Source: CAD feature listing. Evaluate the final solid. Frame: model axes, mm. A direction names the side the tool comes from. Give positions to 0.01 mm unless a question says otherwise; leave off trailing zeros. Order: outer loops, then holes, each group sorted by start corner. A loop starts at its lowest first (then second) coordinate and runs counter-clockwise, first axis right, second up.
from build123d import *

# Parameters (mm, degrees)
ESQUISSE1_W             = 34.9
ESQUISSE1_H             = 3
BOSS_EXTRU_1_DEPTH      = 50
ESQUISSE2_W             = 10
ESQUISSE2_H             = 3.5
BOSS_EXTRU_2_DEPTH      = 9.2
ESQUISSE3_R             = 2.2
BOSS_EXTRU_3_DEPTH      = 4.5
CONG_1_R                = 0.5
ESQUISSE5_W             = 4.7
ESQUISSE5_H             = 2.5
BOSS_EXTRU_5_DEPTH      = 11.8
ENL_V_MAT_EXTRU_1_REACH = 29.05
ESQUISSE6_R             = 1
CONG_2_R                = 10


with BuildPart() as part:
    # Esquisse1 → Boss.-Extru.1 (new body)
    with BuildSketch(Plane.XY):
        with Locations((17.45, 1.5)):
            Rectangle(ESQUISSE1_W, ESQUISSE1_H)
    extrude(amount=BOSS_EXTRU_1_DEPTH)

    # Esquisse2 → Boss.-Extru.2 (add)
    with BuildSketch(Plane(origin=(0, 3, 0), x_dir=(1, 0, 0), z_dir=(0, 1, 0))):
        with Locations((12.1, -8.77)):
            Rectangle(ESQUISSE2_W, ESQUISSE2_H)
    extrude(amount=BOSS_EXTRU_2_DEPTH)

    # Esquisse3 → Boss.-Extru.3 (add)
    with BuildSketch(Plane(origin=(0, 0, 7.02), x_dir=(-1, 0, 0), z_dir=(0, 0, -1))):
        with Locations((-10.6, 8.9)):
            Circle(ESQUISSE3_R)
    extrude(amount=BOSS_EXTRU_3_DEPTH)

    # Congé1
    cong_1_edges = [part.edges().sort_by_distance(p)[0] for p in [
        (12.8, 8.9, 2.52),
    ]]
    fillet(cong_1_edges, radius=CONG_1_R)

    # Esquisse5 → Boss.-Extru.5 (add)
    with BuildSketch(Plane(origin=(0, 3, 0), x_dir=(1, 0, 0), z_dir=(0, 1, 0))):
        with Locations((29.55, -25.8)):
            Rectangle(ESQUISSE5_W, ESQUISSE5_H)
        with Locations((2.35, -25.8)):
            Rectangle(ESQUISSE5_W, ESQUISSE5_H)
    extrude(amount=BOSS_EXTRU_5_DEPTH)

    # Esquisse6 → Enlèv. mat.-Extru.1 (cut, up to next)
    with BuildSketch(Plane.XY.offset(27.05), mode=Mode.PRIVATE) as enl_v_mat_extru_1_sk1:
        with Locations((29.6, 8.9)):
            Circle(ESQUISSE6_R)
    enl_v_mat_extru_1_tool1 = extrude(enl_v_mat_extru_1_sk1.sketch, amount=-ENL_V_MAT_EXTRU_1_REACH, mode=Mode.PRIVATE) & part.part
    add(enl_v_mat_extru_1_tool1.solids().sort_by_distance((29.6, 8.9, 27.05))[0], mode=Mode.SUBTRACT)
    # Esquisse6 → Enlèv. mat.-Extru.1 (cut, up to next)
    with BuildSketch(Plane.XY.offset(27.05), mode=Mode.PRIVATE) as enl_v_mat_extru_1_sk2:
        with Locations((2.3, 8.9)):
            Circle(ESQUISSE6_R)
    enl_v_mat_extru_1_tool2 = extrude(enl_v_mat_extru_1_sk2.sketch, amount=-ENL_V_MAT_EXTRU_1_REACH, mode=Mode.PRIVATE) & part.part
    add(enl_v_mat_extru_1_tool2.solids().sort_by_distance((2.3, 8.9, 27.05))[0], mode=Mode.SUBTRACT)

    # Congé2
    cong_2_edges = [part.edges().sort_by_distance(p)[0] for p in [
        (34.9, 1.5, 50),
        (0, 1.5, 50),
        (34.9, 1.5, 0),
        (0, 1.5, 0),
    ]]
    fillet(cong_2_edges, radius=CONG_2_R)


solid = part.part
(1) Line query: line 1 along X through (y, z) = (13.75, 25); line 2 along Z through (x, y) = (3.5, 12.5); line 3 along Y through (x, z) = (20, 30.5). Output: solid intervals per line, ascending.
(2) Section B-B, the plane z = 4. Return loops of the section in (x, y), plus the area to 3 significant figures.
(3) Section C-C, the plane y = 13.75. Return loops of the section in (x, z), plus the area to 3 significant figures.
(4) Pin query (flat end, axial travel): pin 1 Ø2.5 at (x, y) = (2.3, 8.9) entering from +Z; pin 2 Ø1.7 at (x, y) = (11, 8) entering from -Z; pin 3 Ø8 at (x, y) = (30.5, 10.5) entering from -Z; pin 4 Ø1.8 at (x, y) = (29.6, 8.9) entering from +Z. Return the tip coordinate at first contact, or that it passes through.
(5) Draft query along Y for faces 1 (the cylindrical face through (12.22, 10.39, 5.05)), 2 (the cylindrical face through (3.254, 9.2, 25.818)), 3 (the flat face through (34.9, 1, 25)), 4 (the flat face through (2, 14.8, 26)). Return one class per face: +Y half, -Y half, draft (parallel to the pull), parting line (faces both ways), or undercut.
(6) Section A-A, the plane y = 8.9. Return loops of the section in (x, z).
(7) Section D-D, the plane x = 14. Return loops of the section in (y, z), plus the area to 3 significant figures.
(8) Access query for faces 5 (the flat face through (31.9, 9, 26)), 6 (the flat face through (4.7, 9, 26)), 7 (the cylindrical face through (28.6, 8.9, 25.8)), 8 (the flat face through (28, 9, 27.05)), 9 (the flat face through (7.1, 8, 9)). Directions: +Z, -Z, +X, -X, +Y, -Y. A direction counts if a zero-diameter tool reaches every point of the face in a straight line with its end or side. Return the directions, or none.
Checks:
1. line 1: x = 0 to 4.7, 27.2 to 31.9
1. line 2: z = 24.55 to 27.05
1. line 3: y = 0 to 3
2. outline: (2, 0) - (32.9, 0) - (32.9, 3) - (2, 3) - close; circle Ø4.4 at (10.6, 8.9)
2. area: 108 mm2
3. outline: (0, 24.55) - (4.7, 24.55) - (4.7, 27.05) - (0, 27.05) - close; (27.2, 24.55) - (31.9, 24.55) - (31.9, 27.05) - (27.2, 27.05) - close
3. area: 23.5 mm2
4. pin 1: stops at z = 27.05
4. pin 2: stops at z = 2.52
4. pin 3: stops at z = 24.55
4. pin 4: passes through
5. face 1: undercut
5. face 2: undercut
5. face 3: draft
5. face 4: +Y half
6. outline: (0, 24.55) - (1.3, 24.55) - (1.3, 27.05) - (0, 27.05) - close; (3.3, 24.55) - (4.7, 24.55) - (4.7, 27.05) - (3.3, 27.05) - close; (7.1, 7.02) - (8.4, 7.02) - (8.4, 3.02) arc R0.5 ccw to (8.9, 2.52) - (12.3, 2.52) arc R0.5 ccw to (12.8, 3.02) - (12.8, 7.02) - (17.1, 7.02) - (17.1, 10.52) - (7.1, 10.52) - close; (27.2, 24.55) - (28.6, 24.55) - (28.6, 27.05) - (27.2, 27.05) - close; (30.6, 24.55) - (31.9, 24.55) - (31.9, 27.05) - (30.6, 27.05) - close
7. outline: (0, 0) - (3, 0) - (3, 7.02) - (12.2, 7.02) - (12.2, 10.52) - (3, 10.52) - (3, 50) - (0, 50) - close
7. area: 182 mm2
8. face 5: +Z, -Z, +X, +Y
8. face 6: +Z, -Z, +Y
8. face 7: +Z, -Z
8. face 8: +Z, +X, -X, +Y
8. face 9: +Z, -Z, -X, +Y
